The listing builds one solid part. Answer for the finished solid, in the listing's coordinates (mm). Face numbers are marked on the shaded views. Give positions to 0.01 mm unless a question says otherwise; leave off trailing zeros. Loops run counter-clockwise (first coordinate to the right, second up) from the corner with the lowest first, then second, coordinate; pieces in that order, holes last.
Item 1: The mould has two halves that part along Z. Classify the marked faces 1, 2 and 3: pulls with the +Z half, pulls with the -Z half, needs draft (parallel to the pull), parting line crosses it, or undercut.
Item 2: Section B-B, the plane y = 1.6 is taken. Give the vertices of the cut face in (x, z), and give its area (3 significant figures).
Item 3: Section A-A, the plane x = 0 is taken. Give the vertices of the cut face in (y, z), and give its area (3 significant figures).
Item 4: This flat-tipped pin is pushed along its axis until it touches: pin 1 Ø2.5 at (x, z) = (0, 0) entering from +Y. Where does it stop, or does it pass through?
Item 5: Consider line 1 along Z through (x, y) = (0, 1.3); line 2 along Z through (x, y) = (0.75, 1.6); line 3 along X through (y, z) = (2.4, 3.5). Determine where each line is inside the solid, lowest interval first.
Item 6: Section C-C, the plane z = -1 is taken. Give the vertices of the cut face in (x, y).
Item 7: Section D-D, the plane x = -4 is taken. Give the vertices of the cut face in (y, z), and give its area (3 significant figures).
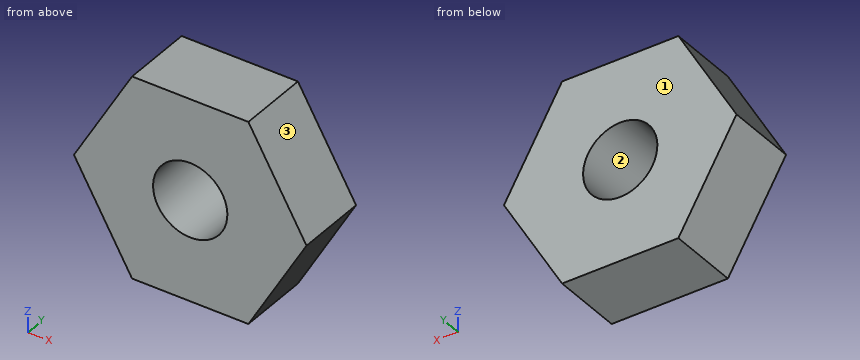
from build123d import *

# Parameters (mm, degrees)
BOSS_EXTRUDE1_DEPTH = 2.7686
SKETCH2_R           = 1.4351
CUT_EXTRUDE2_DEPTH  = 7.558939355


with BuildPart() as part:
    # Sketch1 → Boss-Extrude1 (new body)
    with BuildSketch(Plane(origin=(0, 0, 0), x_dir=(1, 0, 0), z_dir=(0, 1, 0))):
        Polygon((-2.24736479, 3.89255), (-4.494729581, 0), (-2.24736479, -3.89255), (2.24736479, -3.89255), (4.494729581, 0), (2.24736479, 3.89255), align=None)
    extrude(amount=BOSS_EXTRUDE1_DEPTH)

    # Sketch2 → Cut-Extrude2 (cut, through all)
    with BuildSketch(Plane(origin=(0, 0, 0), x_dir=(1, 0, 0), z_dir=(0, 1, 0))):
        with Locations(Location((0, 0, 0), (0, 0, 270))):
            Circle(SKETCH2_R)
    extrude(amount=CUT_EXTRUDE2_DEPTH, mode=Mode.SUBTRACT)


solid = part.part
Worked answers:
1. face 1: needs draft
1. face 2: undercut
1. face 3: pulls with the +Z half
2. outline: (-4.49, 0) - (-2.25, -3.89) - (2.25, -3.89) - (4.49, 0) - (2.25, 3.89) - (-2.25, 3.89) - close; hole circle Ø2.87 at (0, 0)
2. area: 46.0 mm2
3. outline: (0, -3.89) - (2.77, -3.89) - (2.77, -1.44) - (0, -1.44) - close; (0, 1.44) - (2.77, 1.44) - (2.77, 3.89) - (0, 3.89) - close
3. area: 13.6 mm2
4. pin 1: passes through
5. line 1: z = -3.89 to -1.44, 1.44 to 3.89
5. line 2: z = -3.89 to -1.22, 1.22 to 3.89
5. line 3: x = -2.47 to 2.47
6. outline: (-3.92, 0) - (-1.03, 0) - (-1.03, 2.77) - (-3.92, 2.77) - close; (1.03, 0) - (3.92, 0) - (3.92, 2.77) - (1.03, 2.77) - close
7. outline: (0, -0.86) - (2.77, -0.86) - (2.77, 0.86) - (0, 0.86) - close
7. area: 4.74 mm2
